The listing builds one solid part. Answer for the finished solid, in the listing's coordinates (mm). A direction names the side the tool comes from. Coordinates: 2 decimals unless noted, no trailing zeros. Loops run counter-clockwise (first coordinate to the right, second up) from the corner with the lowest first, then second, coordinate; pieces in that order, holes last. Notation, with made-up numbers: M -15.5,-33.75 L 33.5,-33.75 A32 cw 33.5,-1.75 Z; hole C 23.5,-27.5 d4. An arc over 180 degrees is marked long. Answer as a JSON object with one key per item and string values. Group by question number.
1. A cutting plane is placed at B-B on x = -45. Give the vertices of the cut face in (y, z) (3 decimals).
2. For faces 4 (the face through (-45.89, -1.57, 0.95)), 5 (the face through (-29, 0, 0)), determine the directions among +Z, -Z, +X, -X, +Y, -Y from which every point of the face is accessible in a straight line to the end or side of a thin tool.
3. A cutting plane is placed at C-C on y = 4. Give the vertices of the cut face in (x, z) (1 decimal), and give its area (3 significant figures).
4. Determine the mould class of faces 1 (the face through (1.57, 11.19, -0.69)), 2 (the face through (-15, -1, -14.288)), 3 (the face through (2, -2.06, 0.2)) for opening direction Y: released by +Y, released by -Y, zero draft, split by the parting line, or undercut.
5. Given pin 1 (7.5 mm diameter, centred on y = 14.29, z = 0, fed in from -X); pin 2 (3 mm diameter, centred on x = -48.5, z = -11, fed in from +Y), each flat-ended and moving along its own axis, determine where each tip first touches the part or whether it passes through.
6. Straight lines are drawn through the part: L1, parallel to X at y = 7, z = 0 (3 decimals); L2, parallel to Y at x = -4, z = 1.25 (3 decimals); L3, parallel to X at y = -1.5, z = -12.25. For each, find the intervals that lie inside material, in ascending order.
7. A cutting plane is placed at D-D on z = -11.5. Give the vertices of the cut face in (x, y) (3 decimals).
8. A cutting plane is placed at A-A on z = 0. State how many separate pieces and enclosed holes the cut face has, and give its area (3 significant figures).
from build123d import *

# Parameters (mm, degrees)
BASE_FLANGE1_DEPTH = 14.2875
SKETCH6_R          = 3.175
CUT_EXTRUDE1_DEPTH = 66.473550242
SKETCH7_R          = 3.175
CUT_EXTRUDE2_DEPTH = 66.473550242
FILLET2_RADIUS     = 14.2875
FILLET2_LENGTH     = 3.175
FILLET3_RADIUS     = 14.2875
FILLET3_LENGTH     = 3.175


# Sheet-metal steps are written as plain solids
with BuildPart() as part:
    # Sketch1 → Base-Flange1 (new, symmetric)
    with BuildSketch(Plane.XY):
        with BuildLine():
            Line((0, 28.575), (0, 0.7366))
            ThreePointArc((0, 0.7366), (-0.215745145, 0.215745145), (-0.7366, 0))
            Line((-0.7366, 0), (-57.15, 0))
            Line((-57.15, 0), (-57.15, -3.175))
            Line((-57.15, -3.175), (-0.7366, -3.175))
            ThreePointArc((-0.7366, -3.175), (2.029318885, -2.029318885), (3.175, 0.7366))
            Line((3.175, 0.7366), (3.175, 28.575))
            Line((3.175, 28.575), (0, 28.575))
        make_face()
    extrude(amount=BASE_FLANGE1_DEPTH, both=True)

    # Sketch6 → Cut-Extrude1 (cut, through all)
    with BuildSketch(Plane(origin=(0, 0, 0), x_dir=(1, 0, 0), z_dir=(0, 1, 0))):
        with Locations(Location((-42.8625, 0, 0), (0, 0, 180))):
            Circle(SKETCH6_R)
    extrude(amount=-CUT_EXTRUDE1_DEPTH, mode=Mode.SUBTRACT)

    # Sketch7 → Cut-Extrude2 (cut, through all)
    with BuildSketch(Plane.ZY):
        with Locations((0, 14.2875)):
            Circle(SKETCH7_R)
    extrude(amount=-CUT_EXTRUDE2_DEPTH, mode=Mode.SUBTRACT)

    # Fillet2: full round fillet: the end face becomes a half cylinder, R = half its width
    fillet2_face = Plane((-57.15, -1.5875, 0), x_dir=(0, 1, 0), z_dir=(-1, 0, 0))  # on the end face: x along it, z out of the body
    fillet2_slab = fillet2_face.offset(-FILLET2_RADIUS / 2) * Box(FILLET2_LENGTH, 2 * FILLET2_RADIUS, FILLET2_RADIUS, mode=Mode.PRIVATE)  # the body's end, R deep
    fillet2_round = Plane((-42.8625, -1.5875, 0), x_dir=(-1, 0, 0), z_dir=(0, 1, 0)) * Cylinder(FILLET2_RADIUS, FILLET2_LENGTH, mode=Mode.PRIVATE)  # its axis R under the face
    add(fillet2_slab - fillet2_round, mode=Mode.SUBTRACT)

    # Fillet3: full round fillet: the end face becomes a half cylinder, R = half its width
    fillet3_face = Plane((1.5875, 28.575, 0), x_dir=(1, 0, 0), z_dir=(0, 1, 0))  # on the end face: x along it, z out of the body
    fillet3_slab = fillet3_face.offset(-FILLET3_RADIUS / 2) * Box(FILLET3_LENGTH, 2 * FILLET3_RADIUS, FILLET3_RADIUS, mode=Mode.PRIVATE)  # the body's end, R deep
    fillet3_round = Plane((1.5875, 14.2875, 0), x_dir=(0, 1, 0), z_dir=(1, 0, 0)) * Cylinder(FILLET3_RADIUS, FILLET3_LENGTH, mode=Mode.PRIVATE)  # its axis R under the face
    add(fillet3_slab - fillet3_round, mode=Mode.SUBTRACT)


solid = part.part
From the geometry:
{
 "1": {"outline": "M -3.175,-14.127 L 0,-14.127 L 0,-2.348 L -3.175,-2.348 Z; M -3.175,2.348 L 0,2.348 L 0,14.127 L -3.175,14.127 Z"},
 "2": {"face 4": "+Y, -Y", "face 5": "+Z, -Z, -X, +Y"},
 "3": {"outline": "M 0,-14.3 L 3.2,-14.3 L 3.2,14.3 L 0,14.3 Z", "area": "90.7 mm²"},
 "4": {"face 1": "undercut", "face 2": "zero draft", "face 3": "released by -Y"},
 "5": {"pin 1": "stops at x = 0", "pin 2": "stops at y = 0"},
 "6": {"L1": "x = 0 to 3.175", "L2": "y = -3.175 to 0", "L3": "x = -50.22 to 2.47"},
 "7": {"outline": "M -51.341,-3.175 L -0.737,-3.175 A3.912 ccw 3.175,0.737 L 3.175,22.766 L 0,22.766 L 0,0.737 A0.737 cw -0.737,0 L -51.341,0 Z"},
 "8": {"separate pieces": "3", "enclosed holes": "0", "area": "239 mm²"}
}
